Source: CAD feature listing. Evaluate the final solid. Frame: model axes, mm. A direction names the side the tool comes from. Round coordinates to 2 decimals unless told otherwise and drop trailing zeros. Write each loop counter-clockwise with the first axis right and the second up, starting at its lowest first coordinate (ties: lowest second). Pieces come first, ordered by that corner, then holes. Notation, with made-up numbers: M 21.5,67 L 61.5,67 A29 cw 61.5,94 Z; hole C 52.5,39.5 d7. An arc over 180 degrees is marked long. Use a Markdown table: item, result.
```python
from build123d import *

# Parameters (mm, degrees)
SKETCH1_R               = 1.5
BOSS_EXTRUDE1_DEPTH     = 7.62
CUT_EXTRUDE1_DEPTH      = 1.7
CUT_EXTRUDE1_DEPTH_BACK = 1.7
SKETCH2_R               = 1.5
SKETCH3_W               = 34.821950375
SKETCH3_H               = 10.205546921
CUT_EXTRUDE2_DEPTH      = 2.54
FILLET1_R               = 2.54
FILLET2_R               = 2.54


with BuildPart() as part:
    # Sketch1 → Boss-Extrude1 (new body)
    with BuildSketch(Plane(origin=(0, 0, 0), x_dir=(1, 0, 0), z_dir=(0, 1, 0))):
        with BuildLine():
            ThreePointArc((0, 3.175), (-3.175, 0), (0, -3.175))
            Line((0, -3.175), (38.1, -3.175))
            ThreePointArc((38.1, -3.175), (41.275, 0), (38.1, 3.175))
            Line((38.1, 3.175), (0, 3.175))
        make_face()
        with Locations(Location((0, 0, 0), (0, 0, 90))):
            Circle(SKETCH1_R, mode=Mode.SUBTRACT)
        with Locations(Location((38.1, 0, 0), (0, 0, 90))):
            Circle(SKETCH1_R, mode=Mode.SUBTRACT)
    extrude(amount=BOSS_EXTRUDE1_DEPTH)

    # Sketch2 → Cut-Extrude1 (cut, two sides: drawn at the far end of the back side and taken through both)
    with BuildSketch(Plane(origin=(0, 3.81, 0), x_dir=(1, 0, 0), z_dir=(0, 1, 0)).offset(-CUT_EXTRUDE1_DEPTH_BACK)):
        with BuildLine():
            Line((0, 3.175), (5.08, 3.175))
            Line((5.08, 3.175), (5.08, -3.175))
            Line((5.08, -3.175), (0, -3.175))
            ThreePointArc((0, -3.175), (-3.175, 0), (0, 3.175))
        make_face()
        with Locations(Location((0, 0, 0), (0, 0, 90))):
            Circle(SKETCH2_R, mode=Mode.SUBTRACT)
    extrude(amount=CUT_EXTRUDE1_DEPTH + CUT_EXTRUDE1_DEPTH_BACK, mode=Mode.SUBTRACT)

    # Sketch3 → Cut-Extrude2 (cut)
    with BuildSketch(Plane(origin=(0, 7.62, 0), x_dir=(1, 0, 0), z_dir=(0, 1, 0))):
        with Locations((27.570975188, -1.92777346)):
            Rectangle(SKETCH3_W, SKETCH3_H)
    cut_extrude2 = extrude(amount=-CUT_EXTRUDE2_DEPTH, mode=Mode.SUBTRACT)

    # Mirror1: Cut-Extrude2 across plane
    add(cut_extrude2.mirror(Plane.ZX.offset(3.81)), mode=Mode.SUBTRACT)

    # Fillet1
    fillet1_edges = [part.edges().sort_by_distance(p)[0] for p in [
        (10.16, 5.08, 0),
        (10.16, 2.54, 0),
    ]]
    fillet(fillet1_edges, radius=FILLET1_R - 0.0001)  # a hair under: the kernel refuses the full size

    # Fillet2
    fillet2_edges = [part.edges().sort_by_distance(p)[0] for p in [
        (10.16, 7.62, 0),
        (10.16, 0, 0),
    ]]
    fillet(fillet2_edges, radius=FILLET2_R)


solid = part.part
```
Q1. Mould query, pull axis Z, two halves, no side actions, for faces 1 (the cylindrical face through (-0.45, 1.04, -1.43)), 2 (the cylindrical face through (-3.174, 6.55, -0.07)), 3 (the cylindrical face through (-0.45, 6.55, -1.43)), 4 (the flat face through (15, 4, 3.175)). Classes: +Z half, -Z half, draft (parallel to the pull), parting line (faces both ways), or undercut.
Results are:
| item | result |
|---|---|
| face 1 | undercut |
| face 2 | parting line |
| face 3 | undercut |
| face 4 | +Z half |
Q2. Section A-A on y = 4.25. Return loops of the section in (x, z) (3 decimals), plus the area to 3 significant figures.
Results are:
| item | result |
|---|---|
| outline | M 5.08,-3.175 L 38.1,-3.175 A3.175 ccw 38.1,3.175 L 5.08,3.175 Z; hole C 38.1,0 d3 |
| area | 218 mm^2 |
Q3. Reachability of faces 5 (the flat face through (27, 2.54, 0)), 6 (the cylindrical face through (41.274, 3.792, 0.07)), 7 (the flat face through (2, 5.51, 0)), 8 (the flat face through (4, 7.62, 0)), 9 (the flat face through (27, 5.08, 0)) from +Z, -Z, +X, -X, +Y, -Y: full face, straight path, thin tool, end or side. Return the list, or none.
Results are:
| item | result |
|---|---|
| face 5 | +Z, -Z, +X, -Y |
| face 6 | +X, +Y, -Y |
| face 7 | +Z, -Z, -X |
| face 8 | +Z, -Z, +X, -X, +Y |
| face 9 | +Z, -Z, +X, +Y |
Q4. Section C-C on x = 32.5. Return loops of the section in (y, z) (3 decimals).
Results are:
| item | result |
|---|---|
| outline | M 2.54,-3.175 L 5.08,-3.175 L 5.08,3.175 L 2.54,3.175 Z |
Q5. Section B-B on z = 0. Give the number of separate pieces and of enclosed holes in the cut face, plus the area to 3 significant figures.
Results are:
| item | result |
|---|---|
| separate pieces | 4 |
| enclosed holes | 0 |
| area | 134 mm^2 |
Q6. First-contact query: pin 1 Ø3.5 at (y, z) = (4.5, -0.5) entering from -X (3 decimals); pin 2 Ø2.5 at (x, z) = (0, 0) entering from -Y; pin 3 Ø1 at (y, z) = (6, -1) entering from -X; pin 4 Ø3 at (x, z) = (27, -0.5) entering from -Y. Flat tips, straight axial feed; report the tip coordinate or a pass-through.
Results are:
| item | result |
|---|---|
| pin 1 | x = -3.175 |
| pin 2 | through |
| pin 3 | x = -3.14 |
| pin 4 | y = 2.54 |
Q7. Line query: L1, parallel to X at y = 1.25, z = 0.5; L2, parallel to Y at x = 39, z = -2.5; L3, parallel to Y at x = 5, z = -0.75. Output: solid intervals per line, ascending.
Results are:
| item | result |
|---|---|
| L1 | -3.14 to -1.41, 1.41 to 10.49 |
| L2 | 2.54 to 5.08 |
| L3 | 0 to 2.11, 5.51 to 7.62 |
